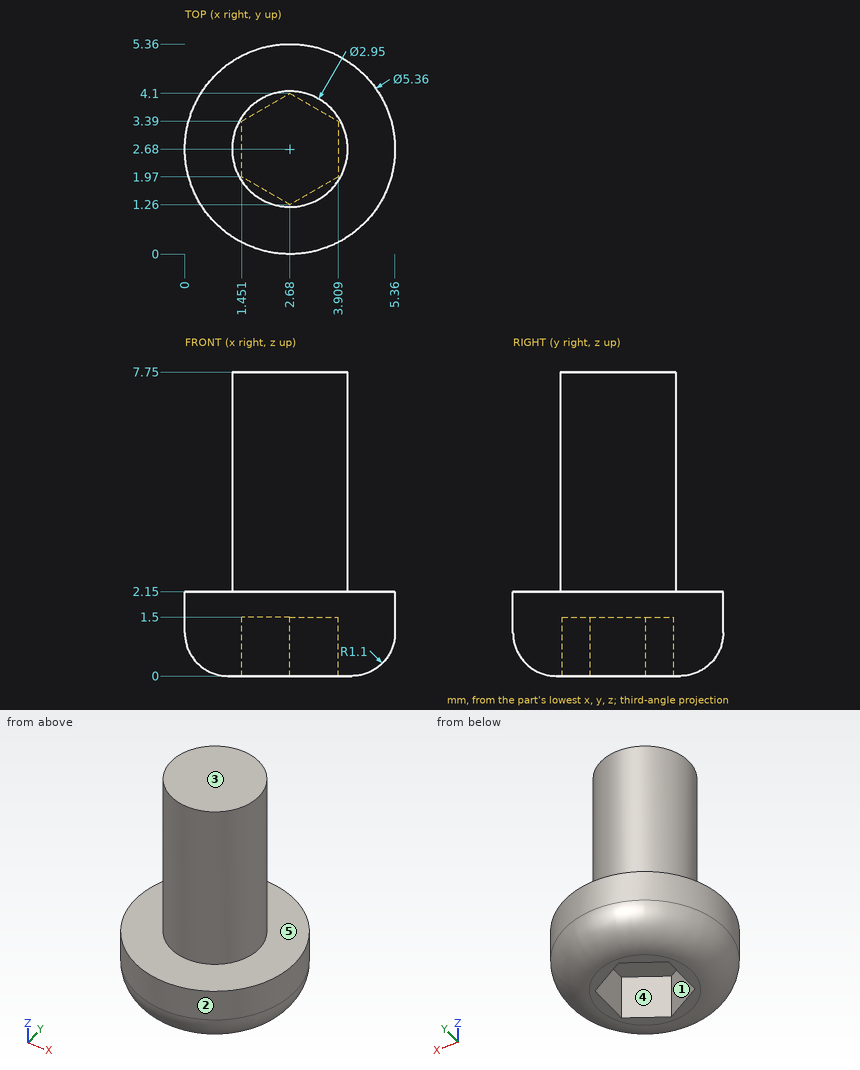
Here's the drawing with two shaded views (mm, measured from the low corner). I have some questions. A direction names the side the tool comes from. Give positions to 0.01 mm unless a question says otherwise; leave off trailing zeros. One line per item, written item: value. Start each with the question number.
Item 1: Which directions (+Z, -Z, +X, -X, +Y, -Y) give clear straight access to the entire face, cutting with the end or side of a thin tool? Please do the marked faces 4 and 5.
Item 2: I'm going to push flat-ended pins straight in: pin 1 (2 mm diameter, centred on y = 4.5, z = 6, fed in from +X) (1 decimal); pin 2 (3 mm diameter, centred on x = 1.5, y = 4, fed in from -Z); pin 3 (2 mm diameter, centred on y = 2.5, z = 6, fed in from +X) (1 decimal); pin 4 (1 mm diameter, centred on x = 4, z = 1.5, fed in from -Y). Where does each tip first touch, or does it pass through?
Item 3: If we mould it in two halves opening along X, with no side actions, what happens to the marked faces 1, 2 and 3? For each: +X half, -X half, draft (parallel to the pull), parting line (faces both ways), or undercut.
Item 4: Please list where these lines run through material, in increasing order: line 1 (Z direction, x = 1.65, y = 2.2); line 2 (X direction, y = 3.6, z = 0.75) (1 decimal); line 3 (Y direction, x = 2.5, z = 0.5) (1 decimal). Write a range as from..to.
Geometry says:
1. face 4: -Z
1. face 5: +Z
2. pin 1: x = 3.9
2. pin 2: z = 0
2. pin 3: x = 4.2
2. pin 4: y = 0.13
3. face 1: undercut
3. face 2: parting line
3. face 3: draft
4. line 1: 1.5..7.75
4. line 2: 0.2..1.8, 3.5..5.1
4. line 3: 0.2..1.4, 4..5.2
